Read the model definition and answer for the solid it produces. Units are mm, in the model's axes. A direction names the side the tool comes from. Give positions to 0.01 mm unless a question says otherwise; leave off trailing zeros. Order: outer loops, then holes, each group sorted by start corner. A loop starts at its lowest first (then second) coordinate and runs counter-clockwise, first axis right, second up. Notation, with made-up numbers: (-1.5, 17) - (7.5, 17) arc R13 ccw to (7.5, 41) - close; hole circle Ø3 at (32, 33). An arc over 180 degrees is marked (long way). Write each question's results on one line, items separated by ' | '.
from build123d import *

# Parameters (mm, degrees)
PAD_DEPTH = 0.9


with BuildPart() as part:
    # Sketch → Pad (new body, symmetric)
    with BuildSketch(Plane.XZ):
        Polygon((-3.3, 0), (3.3, 0), (2.5, 1), (2.5, 5), (2, 5), (2, 10), (-2, 10), (-2, 5), (-2.5, 5), (-2.5, 1), align=None)
    extrude(amount=PAD_DEPTH, both=True)


solid = part.part
(1) Consider probe 1 along X at (y, z) = (-0.65, 4.5); probe 2 along X at (y, z) = (0.1, 6.5); probe 3 along Z at (x, y) = (3, 0.2) (3 decimals). Determine where each line is inside the solid, lowest interval first. Write a range as [from, to].
Conclusion:
probe 1: [-2.5, 2.5] | probe 2: [-2, 2] | probe 3: [0, 0.375]
(2) Each of these flat-tipped pins is pushed along its axis until it touches: pin 1 (0.6 mm diameter, centred on x = -2.5, y = 0, fed in from +Z); pin 2 (0.9 mm diameter, centred on y = 0, z = 6.5, fed in from -X); pin 3 (0.9 mm diameter, centred on y = 0, z = 7, fed in from +X). Where does it stop, or does it pass through?
Conclusion:
pin 1: z = 5 | pin 2: x = -2 | pin 3: x = 2
(3) For faces 1 (the face through (2, 0, 7)), 2 (the face through (0, -0.9, 5)), 3 (the face through (-2.5, 0, 3)), determine the directions among +Z, -Z, +X, -X, +Y, -Y from which every point of the face is accessible in a straight line to the end or side of a thin tool.
Conclusion:
face 1: +Z, +X, +Y, -Y | face 2: +Z, -Z, +X, -X, -Y | face 3: +Z, -X, +Y, -Y
(4) Section A-A (y = 0.6) is taken. Give the vertices of the cut face in (x, z).
Conclusion:
outline: (-3.3, 0) - (3.3, 0) - (2.5, 1) - (2.5, 5) - (2, 5) - (2, 10) - (-2, 10) - (-2, 5) - (-2.5, 5) - (-2.5, 1) - close
(5) Section C-C (z = 5.5) is taken. Give the vertices of the cut face in (x, y).
Conclusion:
outline: (-2, -0.9) - (2, -0.9) - (2, 0.9) - (-2, 0.9) - close
(6) Section B-B (z = 4.5) is taken. Give the vertices of the cut face in (x, y).
Conclusion:
outline: (-2.5, -0.9) - (2.5, -0.9) - (2.5, 0.9) - (-2.5, 0.9) - close
